from build123d import *

# Parameters (mm, degrees)
SKETCH_1_W          = 112.3
SKETCH_1_H          = 95
EXTRUDE_1_DEPTH     = 120
SKETCH_2_W          = 72.3
SKETCH_2_H          = 22
CUT_EXTRUDE_1_DEPTH = 190.832268068
CUT_EXTRUDE_2_DEPTH = 25
SKETCH_4_R          = 3.25
CUT_EXTRUDE_3_DEPTH = 25
SKETCH_6_W          = 22
SKETCH_6_H          = 95
CUT_EXTRUDE_4_DEPTH = 15


with BuildPart() as part:
    # 草图1 → 凸台-拉伸1 (new body)
    with BuildSketch(Plane.XY):
        with Locations((56.15, 47.5)):
            Rectangle(SKETCH_1_W, SKETCH_1_H)
    extrude(amount=EXTRUDE_1_DEPTH)

    # 草图2 → 切除-拉伸1 (cut, through all)
    with BuildSketch(Plane.XZ):
        with Locations((56.15, 109)):
            Rectangle(SKETCH_2_W, SKETCH_2_H)
        with Locations((56.15, 11)):
            Rectangle(SKETCH_2_W, SKETCH_2_H)
    extrude(amount=-CUT_EXTRUDE_1_DEPTH, mode=Mode.SUBTRACT)

    # 草图3 → 切除-拉伸2 (cut)
    with BuildSketch(Plane.ZY):
        with BuildLine():
            Line((106.7, 18.576960217), (106.7, 78.576960217))
            ThreePointArc((106.7, 78.576960217), (110, 81.876960217), (113.3, 78.576960217))
            Line((113.3, 78.576960217), (113.3, 18.576960217))
            ThreePointArc((113.3, 18.576960217), (110, 15.276960217), (106.7, 18.576960217))
        make_face()
        with BuildLine():
            Line((13.3, 18.576960217), (13.3, 78.576960217))
            ThreePointArc((13.3, 78.576960217), (10, 81.876960217), (6.7, 78.576960217))
            Line((6.7, 78.576960217), (6.7, 18.576960217))
            ThreePointArc((6.7, 18.576960217), (10, 15.276960217), (13.3, 18.576960217))
        make_face()
    extrude(amount=-CUT_EXTRUDE_2_DEPTH, mode=Mode.SUBTRACT)

    # 草图4 → 切除-拉伸3 (cut)
    with BuildSketch(Plane(origin=(112.3, 0, 0), x_dir=(0, 0, -1), z_dir=(1, 0, 0))):
        with Locations((-110, 82.5)):
            Circle(SKETCH_4_R)
        with Locations((-10, 82.5)):
            Circle(SKETCH_4_R)
        with Locations((-10, 12.5)):
            Circle(SKETCH_4_R)
        with Locations((-110, 12.5)):
            Circle(SKETCH_4_R)
    extrude(amount=-CUT_EXTRUDE_3_DEPTH, mode=Mode.SUBTRACT)

    # 草图6 → 切除-拉伸4 (cut)
    with BuildSketch(Plane(origin=(112.3, 0, 0), x_dir=(0, 0, -1), z_dir=(1, 0, 0))):
        with Locations((-60, 47.5)):
            Rectangle(SKETCH_6_W, SKETCH_6_H)
    extrude(amount=-CUT_EXTRUDE_4_DEPTH, mode=Mode.SUBTRACT)


solid = part.part
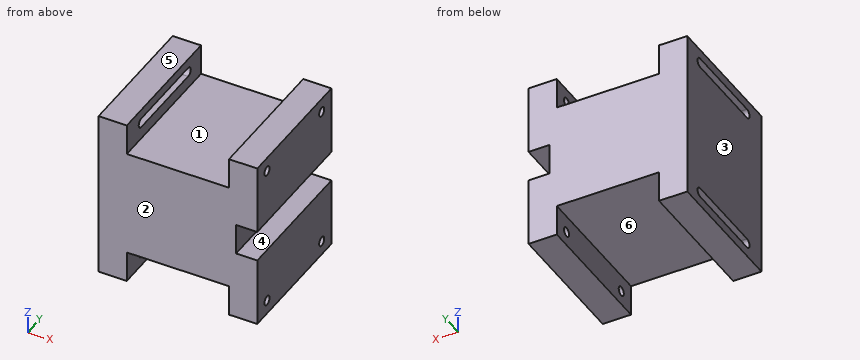
Check sheet for the modelled part. Datum: model origin and axes. Units: mm. Face numbers are marked on the shaded views. A direction names the side the tool comes from. Coordinates: 2 decimals unless noted, no trailing zeros. Write each loop counter-clockwise with the first axis right and the second up, starting at its lowest first coordinate (ties: lowest second). Pieces come first, ordered by that corner, then holes. Notation, with made-up numbers: M -36,34.5 L -12,34.5 A20 ccw -12,45.5 Z; hole C 49,53.5 d4. An arc over 180 degrees is marked long. Answer as CSV lines item,"result".
Q1. Cross-section at D-D (y = 12.5). Record the boundary of the cut face in (x, z).
Check result:
outline,"M 0,0 L 20,0 L 20,22 L 92.3,22 L 92.3,13.25 L 112.3,13.25 L 112.3,49 L 97.3,49 L 97.3,71 L 112.3,71 L 112.3,106.75 L 92.3,106.75 L 92.3,98 L 20,98 L 20,120 L 0,120 Z; M 92.3,0 L 112.3,0 L 112.3,6.75 L 92.3,6.75 Z; M 92.3,113.25 L 112.3,113.25 L 112.3,120 L 92.3,120 Z"
Q2. Go/stop test with flat-tipped pins: pin 1 (5 mm diameter, centred on y = 12.5, z = 10, fed in from +X); pin 2 (21.5 mm diameter, centred on x = 40.5, y = 71, fed in from -Z); pin 3 (1.5 mm diameter, centred on x = 56.5, y = 54, fed in from +Z). Record where each tip stops, or that it passes through.
Check result:
pin 1,"x = 20"
pin 2,"z = 22"
pin 3,"z = 98"
Q3. Cross-section at A-A (y = 67). Record the boundary of the cut face in (x, z).
Check result:
outline,"M 0,0 L 20,0 L 20,6.7 L 0,6.7 Z; M 0,13.3 L 20,13.3 L 20,22 L 92.3,22 L 92.3,0 L 112.3,0 L 112.3,49 L 97.3,49 L 97.3,71 L 112.3,71 L 112.3,120 L 92.3,120 L 92.3,98 L 20,98 L 20,106.7 L 0,106.7 Z; M 0,113.3 L 20,113.3 L 20,120 L 0,120 Z"
Q4. Set-up check for the marked faces 4, 5 and 6: record each of +Z, -Z, +X, -X, +Y, -Y from which the full face is reachable in a straight line by a thin tool's end or side.
Check result:
face 4,"+X, +Y, -Y"
face 5,"+Z, +X, -X, +Y, -Y"
face 6,"-Z, +Y, -Y"
Q5. Cross-section at B-B (z = 10). Record the boundary of the cut face in (x, y), then the cut area to 3 significant figures.
Check result:
outline,"M 0,0 L 20,0 L 20,15.28 L 0,15.28 Z; M 0,81.88 L 20,81.88 L 20,95 L 0,95 Z; M 92.3,0 L 112.3,0 L 112.3,9.25 L 92.3,9.25 Z; M 92.3,15.75 L 112.3,15.75 L 112.3,79.25 L 92.3,79.25 Z; M 92.3,85.75 L 112.3,85.75 L 112.3,95 L 92.3,95 Z"
area,"2,210 mm^2"
Q6. Cross-section at C-C (z = 100). Record the boundary of the cut face in (x, y).
Check result:
outline,"M 0,0 L 20,0 L 20,95 L 0,95 Z; M 92.3,0 L 112.3,0 L 112.3,95 L 92.3,95 Z"
Q7. Mould release check, pull along X, two halves, no side actions. Record for the marked faces 1, 2 and 3: released by +X, released by -X, zero draft, split by the parting line, or undercut.
Check result:
face 1,"undercut"
face 2,"zero draft"
face 3,"released by -X"
Q8. Material ranges on probe 1 along Z at (x, y) = (6, 23); probe 2 along Y at (x, z) = (102, 10); probe 3 along Z at (x, y) = (103, 12), recorded low to high. Write a range as from..to.
Check result:
probe 1,"0..6.7, 13.3..106.7, 113.3..120"
probe 2,"0..9.25, 15.75..79.25, 85.75..95"
probe 3,"0..6.79, 13.21..49, 71..106.79, 113.21..120"
